Design review of the part built by this model. Coordinates are the model's own, in mm. A direction names the side the tool comes from. Coordinates: 2 decimals unless noted, no trailing zeros. Loops run counter-clockwise (first coordinate to the right, second up) from the corner with the lowest first, then second, coordinate; pieces in that order, holes last.
from build123d import *

# Parameters (mm, degrees)
ESBO_O1_W                = 60
ESBO_O1_H                = 20
RESSALTO_EXTRUS_O1_DEPTH = 20
ESBO_O2_W                = 40
ESBO_O2_H                = 20
RESSALTO_EXTRUS_O2_DEPTH = 20
ESBO_O3_W                = 20
ESBO_O3_H                = 20
RESSALTO_EXTRUS_O3_DEPTH = 20


with BuildPart() as part:
    # Esboço1 → Ressalto-extrusão1 (new body)
    with BuildSketch(Plane.XY):
        with Locations((30, 10)):
            Rectangle(ESBO_O1_W, ESBO_O1_H)
    extrude(amount=RESSALTO_EXTRUS_O1_DEPTH)

    # Esboço2 → Ressalto-extrusão2 (add)
    with BuildSketch(Plane.XY.offset(20)):
        with Locations((40, 10)):
            Rectangle(ESBO_O2_W, ESBO_O2_H)
    extrude(amount=RESSALTO_EXTRUS_O2_DEPTH)

    # Esboço3 → Ressalto-extrusão3 (add)
    with BuildSketch(Plane(origin=(0, 20, 0), x_dir=(1, 0, 0), z_dir=(0, 1, 0))):
        with Locations((50, -10)):
            Rectangle(ESBO_O3_W, ESBO_O3_H)
    extrude(amount=RESSALTO_EXTRUS_O3_DEPTH)


solid = part.part
Q1. Take a section at A-A, the plane z = 8.5. Write out the cut boundary in (x, y), then the cut area to 3 significant figures.
Q2. Take a section at C-C, the plane x = 6. Write out the cut boundary in (y, z), then the cut area to 3 significant figures.
Q3. Take a section at B-B, the plane y = 19. Write out the cut boundary in (x, z).
Q4. Clearance check with a flat-ended pin moving along its axis: pin 1 Ø10 at (y, z) = (28, 14) entering from -X. State where the tip first meets the part, or that it passes through.
Q5. Machinability: for faces 1 (the flat face through (60, 15, 16)), 2 (the flat face through (50, 30, 20)), 3 (the flat face through (40, 30, 10)), 4 (the flat face through (50, 40, 10)), 5 (the flat face through (10, 10, 20)), which of the approach directions +Z, -Z, +X, -X, +Y, -Y give a long, thin tool a straight path to every point of the face, cutting with its end or side? Answer none if there is none.
Q6. Take a section at D-D, the plane x = 39. Write out the cut boundary in (y, z), then the cut area to 3 significant figures.
Q7. For line 1 (X direction, y = 12, z = 24); line 2 (Y direction, x = 57, z = 27.5), list the stretches that pass through material, from the lowest coordinate up.
Entries:
1. outline: (0, 0) - (60, 0) - (60, 40) - (40, 40) - (40, 20) - (0, 20) - close
1. area: 1,600 mm2
2. outline: (0, 0) - (20, 0) - (20, 20) - (0, 20) - close
2. area: 400 mm2
3. outline: (0, 0) - (60, 0) - (60, 40) - (20, 40) - (20, 20) - (0, 20) - close
4. pin 1: stops at x = 40
5. face 1: +Z, -Z, +X, +Y, -Y
5. face 2: +Z, +X, -X, +Y
5. face 3: +Z, -Z, -X, +Y
5. face 4: +Z, -Z, +X, -X, +Y
5. face 5: +Z, -X, +Y, -Y
6. outline: (0, 0) - (20, 0) - (20, 40) - (0, 40) - close
6. area: 800 mm2
7. line 1: x = 20 to 60
7. line 2: y = 0 to 20
